from build123d import *

# Parameters (mm, degrees)
SKETCH1_W           = 151
SKETCH1_H           = 95
BOSS_EXTRUDE1_DEPTH = 65
BOSS_EXTRUDE2_DEPTH = 65
CUT_EXTRUDE1_REACH  = 143
SKETCH3_W           = 5
SKETCH3_H           = 7.5
SKETCH3_W_2         = 40
SHELL1_T            = -1


with BuildPart() as part:
    # Sketch1 → Boss-Extrude1 (new body)
    with BuildSketch(Plane.XY):
        Rectangle(SKETCH1_W, SKETCH1_H)
    extrude(amount=-BOSS_EXTRUDE1_DEPTH)

    # Sketch2 → Boss-Extrude2 (add)
    with BuildSketch(Plane.XY):
        Polygon((-65.5, 47.5), (-65.5, 55), (-55.5, 55), (-55.5, 52.5), (-63, 52.5), (-63, 47.5), align=None)
    extrude(amount=-BOSS_EXTRUDE2_DEPTH)

    # Sketch3 → Cut-Extrude1 (cut, up to next)
    with BuildSketch(Plane.ZY.offset(65.5), mode=Mode.PRIVATE) as cut_extrude1_sk1:
        with Locations((-62.5, 51.25)):
            Rectangle(SKETCH3_W, SKETCH3_H)
    cut_extrude1_tool1 = extrude(cut_extrude1_sk1.sketch, amount=-CUT_EXTRUDE1_REACH, mode=Mode.PRIVATE) & part.part
    add(cut_extrude1_tool1.solids().sort_by_distance((-65.5, 51.25, -62.5))[0], mode=Mode.SUBTRACT)
    # Sketch3 → Cut-Extrude1 (cut, up to next)
    with BuildSketch(Plane.ZY.offset(65.5), mode=Mode.PRIVATE) as cut_extrude1_sk2:
        with Locations((-32.5, 51.25)):
            Rectangle(SKETCH3_W_2, SKETCH3_H)
    cut_extrude1_tool2 = extrude(cut_extrude1_sk2.sketch, amount=-CUT_EXTRUDE1_REACH, mode=Mode.PRIVATE) & part.part
    add(cut_extrude1_tool2.solids().sort_by_distance((-65.5, 51.25, -32.5))[0], mode=Mode.SUBTRACT)
    # Sketch3 → Cut-Extrude1 (cut, up to next)
    with BuildSketch(Plane.ZY.offset(65.5), mode=Mode.PRIVATE) as cut_extrude1_sk3:
        with Locations((-2.5, 51.25)):
            Rectangle(SKETCH3_W, SKETCH3_H)
    cut_extrude1_tool3 = extrude(cut_extrude1_sk3.sketch, amount=-CUT_EXTRUDE1_REACH, mode=Mode.PRIVATE) & part.part
    add(cut_extrude1_tool3.solids().sort_by_distance((-65.5, 51.25, -2.5))[0], mode=Mode.SUBTRACT)

    # Shell1
    shell1_openings = [part.faces().sort_by_distance(p)[0] for p in [
        (0, -47.5, -32.5),
    ]]
    offset(amount=SHELL1_T, openings=shell1_openings, kind=Kind.INTERSECTION)


solid = part.part
Source: CAD feature listing. Evaluate the final solid. Frame: model axes, mm. A direction names the side the tool comes from. Give positions to 0.01 mm unless a question says otherwise; leave off trailing zeros. Loops run counter-clockwise (first coordinate to the right, second up) from the corner with the lowest first, then second, coordinate; pieces in that order, holes last. Notation, with made-up numbers: (41, 88) -> (92, 88) arc R14 ccw to (92, 103) -> close; hole circle Ø2 at (23, -35.75). An arc over 180 degrees is marked (long way). Use a Markdown table: item, result. Add a question column.
1) Pull-direction query (Z, two-part tool) for faces 1 (the face through (-62, 53, -12.5)), 2 (the face through (75.5, -1, -32)); classes: +Z half, -Z half, draft (parallel to the pull), parting line (faces both ways), or undercut.
2) Reachability of faces 3 (the face through (-60, 53.5, -56)), 4 (the face through (-1, 0, -1)), 5 (the face through (-63, 50, -9)), 6 (the face through (-62, 53, -52.5)) from +Z, -Z, +X, -X, +Y, -Y: full face, straight path, thin tool, end or side. Return the list, or none.
3) Section query C-C, the plane z = -34. Return the cut outline in (x, y), then the cut area to 3 significant figures.
4) First-contact query: pin 1 (1.5 mm diameter, centred on x = 27, z = -43, fed in from +Y); pin 2 (1.6 mm diameter, centred on y = 51.5, z = -10, fed in from +X); pin 3 (8 mm diameter, centred on x = -63, y = 53, fed in from -Z). Flat tips, straight axial feed; report the tip coordinate or a pass-through.
5) Section query A-A, the plane y = 22. Return the cut outline in (x, z), then the cut area to 3 significant figures.
6) Section query B-B, the plane x = 31. Return the cut outline in (y, z).
7) Line query: line 1 along Z through (x, y) = (-51, -5); line 2 along X through (y, z) = (-13.5, -18); line 3 along Y through (x, z) = (31, -43). Output: solid intervals per line, ascending. Write a range as [from, to].
Numbers:
| question | item | result |
|---|---|---|
| 1 | face 1 | undercut |
| 1 | face 2 | draft |
| 2 | face 3 | none |
| 2 | face 4 | -Y |
| 2 | face 5 | +Z, -Z, +X |
| 2 | face 6 | +X, -X, +Y |
| 3 | outline | (-75.5, -47.5) -> (-74.5, -47.5) -> (-74.5, 46.5) -> (74.5, 46.5) -> (74.5, -47.5) -> (75.5, -47.5) -> (75.5, 47.5) -> (-75.5, 47.5) -> close |
| 3 | area | 339 mm2 |
| 4 | pin 1 | stops at y = 47.5 |
| 4 | pin 2 | stops at x = -63 |
| 4 | pin 3 | stops at z = -60 |
| 5 | outline | (-75.5, -65) -> (75.5, -65) -> (75.5, 0) -> (-75.5, 0) -> close; hole (-74.5, -64) -> (74.5, -64) -> (74.5, -1) -> (-74.5, -1) -> close |
| 5 | area | 428 mm2 |
| 6 | outline | (-47.5, -65) -> (47.5, -65) -> (47.5, 0) -> (-47.5, 0) -> (-47.5, -1) -> (46.5, -1) -> (46.5, -64) -> (-47.5, -64) -> close |
| 7 | line 1 | z = [-65, -64], [-1, 0] |
| 7 | line 2 | x = [-75.5, -74.5], [74.5, 75.5] |
| 7 | line 3 | y = [46.5, 47.5] |
